Design review of the part built by this model. Coordinates are the model's own, in mm. A direction names the side the tool comes from. Round coordinates to 2 decimals unless told otherwise and drop trailing zeros. Order: outer loops, then holes, each group sorted by start corner. A loop starts at its lowest first (then second) coordinate and runs counter-clockwise, first axis right, second up. Notation, with made-up numbers: (84, 16) - (128, 16) arc R22 ccw to (128, 37) - close; hole circle Ø8 at (65.5, 1). An arc over 180 degrees is marked (long way). Write item = value, one per line.
from build123d import *

# Parameters (mm, degrees)
F0_R     = 2.5
F1_DEPTH = 5
F0_R_2   = 4
F2_DEPTH = 1
F3_R     = 0.99999


# Not quite as in the source:
# - a fillet or chamfer is up to 0.001 mm smaller than in the source, because OpenCascade refuses the exact size


with BuildPart() as f1:
    # F0 (on Top) → F1 (new body)
    with BuildSketch(Plane.XY):
        Circle(F0_R)
    extrude(amount=F1_DEPTH)

    # F0 (on Top) → F2 (join)
    with BuildSketch(Plane.XY):
        Circle(F0_R_2)
        Circle(F0_R, mode=Mode.SUBTRACT)
    extrude(amount=F2_DEPTH)

    # F3 (radius 1 in the source; OpenCascade refuses exactly that, so slightly less here)
    f3_edges = [f1.edges().sort_by_distance(p)[0] for p in [
        (-4, 0, 0),
        (-2.5, 0, 5),
    ]]
    fillet(f3_edges, radius=F3_R)


solid = f1.part
1) To check wall thickness, follow L1, parallel to Y at x = 0, z = 3.9; L2, parallel to Z at x = -2.5, y = 0.75; L3, parallel to Y at x = 3.5, z = 0.6. State the ranges of each line that lie inside material, in increasing order. Write a range as from..to.
Findings:
L1 = -2.5..2.5
L2 = 0..1
L3 = -1.76..1.76
2) Clearance check with flat-ended pins moving along their axes: pin 1 Ø2 at (x, y) = (3, 1) entering from +Z; pin 2 Ø1 at (x, z) = (-0.5, 3.5) entering from +Y; pin 3 Ø3 at (x, y) = (-1, -1.5) entering from -Z. State where each tip first meets the part, or that it passes through.
Findings:
pin_1 = 4.75
pin_2 = 2.5
pin_3 = 0
3) For faces 1 (the flat face through (0, 0, 5)), 2 (the flat face through (2, 2, 1)), list the 3-axis set-ups (+Z, -Z, +X, -X, +Y, -Y) from which the entire face can be reached by the end or side of a thin tool; tool diameter is ignored.
Findings:
face_1 = +Z, +X, -X, +Y, -Y
face_2 = +Z
4) We need section D-D on z = 0.3. Write out the cut boundary in (x, y), and give its area (3 significant figures).
Findings:
outline = circle Ø7.43 at (0, 0)
area = 43.3 mm^2
5) We need section C-C on z = 1.55. Write out the cut boundary in (x, y), and give its area (3 significant figures).
Findings:
outline = circle Ø5 at (0, 0)
area = 19.6 mm^2
